Can you work these out from the model? Positions are in its coordinate system, mm. Round coordinates to 2 decimals unless told otherwise and drop trailing zeros. Loops run counter-clockwise (first coordinate to the right, second up) from the corner with the lowest first, then second, coordinate; pieces in that order, holes last. Notation, with made-up numbers: (-7, 79) -> (10, 79) arc R16 ccw to (10, 93) -> close; hole circle Ø1 at (80, 38). An arc over 180 degrees is marked (long way). Write item = value, one per line.
from build123d import *

# Parameters (mm, degrees)
CYLINDER001_R       = 14
CYLINDER001_DEPTH   = 19
BOX_W               = 17.5
BOX_H               = 14.5
BOX_DEPTH           = 16.3
CUT_PLACEMENT_ANGLE = -90


with BuildPart() as cylinder001:
    # Cylinder001 → Cylinder001 (new body)
    with BuildSketch(Plane.XY):
        Circle(CYLINDER001_R)
    extrude(amount=CYLINDER001_DEPTH)


with BuildPart() as cut:
    # Box → Box (new body)
    with BuildSketch(Plane(origin=(0, -7.25, 2.7), x_dir=(1, 0, 0), z_dir=(0, 0, 1))):
        with Locations((8.75, 7.25)):
            Rectangle(BOX_W, BOX_H)
    extrude(amount=BOX_DEPTH)

    # Cut: cut Cylinder001
    add(cylinder001.part, mode=Mode.SUBTRACT)


with BuildPart() as cut_1:
    # Cut placement: moved
    add(cut.part.rotate(Axis((0, 0, 0), (0, 0, 1)), CUT_PLACEMENT_ANGLE))


solid = cut_1.part
1. I need wall thicknesses on line 1 (Y direction, x = 0.25, z = 18.75); line 2 (X direction, y = -13, z = 12.5); line 3 (Y direction, x = -6.25, z = 17.5). Which ranges of each line are inside material? Lowest first, please. Write a range as [from, to].
Entries:
line_1 = [-17.5, -14]
line_2 = [-7.25, -5.2], [5.2, 7.25]
line_3 = [-17.5, -12.53]
2. Suppose I cut it at A-A, the plane y = -12.4. List the corners of the cut face in (x, z) for me, and give its area (3 significant figures).
Entries:
outline = (-7.25, 2.7) -> (-6.5, 2.7) -> (-6.5, 19) -> (-7.25, 19) -> close; (6.5, 2.7) -> (7.25, 2.7) -> (7.25, 19) -> (6.5, 19) -> close
area = 24.5 mm²
3. Suppose I cut it at B-B, the plane x = 0. List the corners of the cut face in (y, z) for me, and give its area (4 significant figures).
Entries:
outline = (-17.5, 2.7) -> (-14, 2.7) -> (-14, 19) -> (-17.5, 19) -> close
area = 57.05 mm²
4. We'd pull the mould along X, two halves only. Please class faces 1 (the cylindrical face through (0, -14, 11)), 2 (the flat face through (7.25, -15, 11)), 3 (the flat face through (-7.25, -15, 11)), 4 (the flat face through (0, -15, 19)): released by +X, released by -X, zero draft, split by the parting line, or undercut.
Entries:
face_1 = undercut
face_2 = released by +X
face_3 = released by -X
face_4 = zero draft
5. Suppose I cut it at C-C, the plane z = 11. List the corners of the cut face in (x, y) for me, and give its area (3 significant figures).
Entries:
outline = (-7.25, -17.5) -> (7.25, -17.5) -> (7.25, -11.98) arc R14 cw to (-7.25, -11.98) -> close
area = 60.2 mm²
